from build123d import *

# Parameters (mm, degrees)
SKETCH1_W                  = 12.7
SKETCH1_H                  = 12.7
BOSS_EXTRUDE1_DEPTH        = 31.75
F_10_32_TAPPED_HOLE1_D     = 4.0386
F_10_32_TAPPED_HOLE1_DEPTH = 11.938
F_10_32_TAPPED_HOLE1_TIP   = 1.213317848
M3X0_5_TAPPED_HOLE1_D      = 2.5


with BuildPart() as part:
    # Sketch1 → Boss-Extrude1 (new body)
    with BuildSketch(Plane(origin=(0, 0, 0), x_dir=(0, 0, -1), z_dir=(1, 0, 0))):
        with Locations((6.35, 6.35)):
            Rectangle(SKETCH1_W, SKETCH1_H)
    extrude(amount=BOSS_EXTRUDE1_DEPTH)

    # #10-32 Tapped Hole1
    with Locations(Plane(origin=(31.75, 0.23991288, -27.515191368), x_dir=(0, 0, 1), z_dir=(1, 0, 0))):
        with Locations((21.165191368, -6.11008712)):
            Hole(F_10_32_TAPPED_HOLE1_D / 2, depth=F_10_32_TAPPED_HOLE1_DEPTH)
            with Locations((0, 0, -(F_10_32_TAPPED_HOLE1_DEPTH + F_10_32_TAPPED_HOLE1_TIP / 2))):  # 118° drill point
                Cone(0, F_10_32_TAPPED_HOLE1_D / 2, F_10_32_TAPPED_HOLE1_TIP, mode=Mode.SUBTRACT)

    # M3x0.5 Tapped Hole1 (through all)
    with Locations(Plane(origin=(0.397447268, 0, -0.674798578), x_dir=(1, 0, 0), z_dir=(0, -1, 0))):
        with Locations((7.476552732, -5.495536137)):
            Hole(M3X0_5_TAPPED_HOLE1_D / 2)


solid = part.part
Here's how the part is built. I have some questions about the finished solid (model axes, mm). A direction names the side the tool comes from. Coordinates: 2 decimals unless noted, no trailing zeros. Use one line per item in the form item = value.
1) I need wall thicknesses on line 1 (Y direction, x = 23, z = -6.35); line 2 (X direction, y = 3.5, z = -6.5); line 3 (X direction, y = 6, z = -8). Which ranges of each line are inside material? Lowest first, please.
Solved:
line_1 = 0 to 4.33, 8.37 to 12.7
line_2 = 0 to 6.67, 9.08 to 31.75
line_3 = 0 to 19.61
2) On a 3-axis mill with a long thin cutter (end or side, diameter ignored), from which of +Z, -Z, +X, -X, +Y, -Y can I reach the whole of each face in a straight line? I mean faces 4 (the cylindrical face through (25.7, 4.65, -7.44)), 5 (the flat face through (16, 0, -6)). Say none if no direction works.
Solved:
face_4 = +X
face_5 = +Z, -Z, +X, -X, -Y
3) Thinking about a two-plate mould opening in Z: for faces 1 (the cylindrical face through (9.123, 6.439, -6.115)), 2 (the flat face through (16, 6, -12.7)), 3 (the flat face through (16, 12.7, -6)), which applies, released by +Z, released by -Z, zero draft, split by the parting line, or undercut?
Solved:
face_1 = undercut
face_2 = released by -Z
face_3 = zero draft
